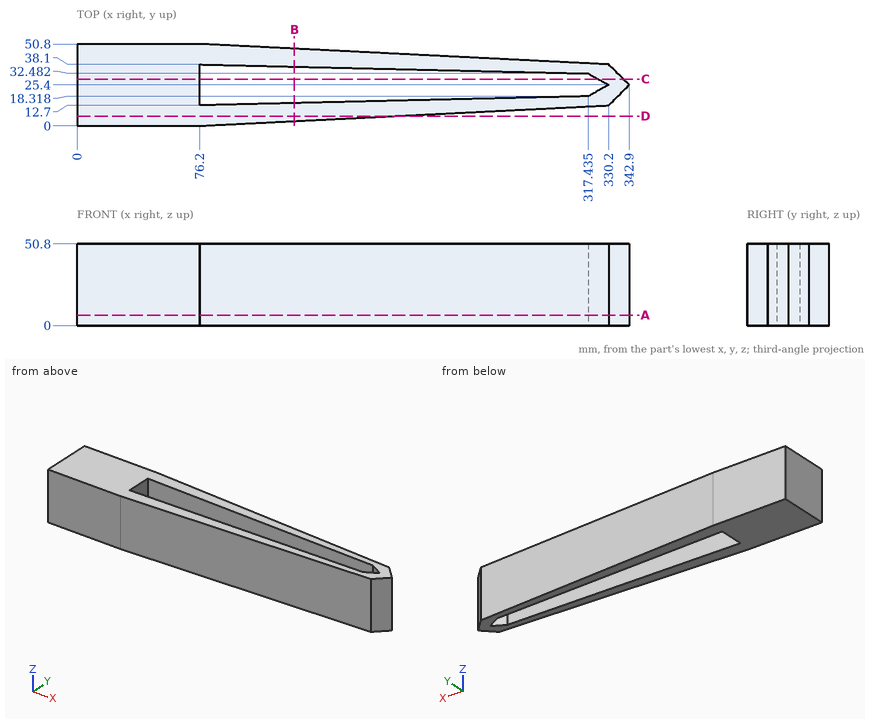
Check sheet for the drawn part. Datum: minimum x, y, z corner. Units: mm. Give positions to 0.01 mm unless a question says otherwise; leave off trailing zeros. Order: outer loops, then holes, each group sorted by start corner. A loop starts at its lowest first (then second) coordinate and runs counter-clockwise, first axis right, second up. Notation, with made-up numbers: (-38.75, 2.5) - (7.25, 2.5) arc R26 ccw to (7.25, 38.5) - close; hole circle Ø5 at (71, 44.5). An arc over 180 degrees is marked (long way). Answer as a JSON object with one key per item and string values.
(1) Cross-section at D-D (y = 6). Record the cut outline in (x, z).
Report:
{"outline": "(0, 0) - (196.2, 0) - (196.2, 50.8) - (0, 50.8) - close"}
(2) Cross-section at C-C (y = 29). Record the cut outline in (x, z).
Report:
{"outline": "(0, 0) - (76.2, 0) - (76.2, 50.8) - (0, 50.8) - close; (323.71, 0) - (339.3, 0) - (339.3, 50.8) - (323.71, 50.8) - close"}
(3) Cross-section at A-A (z = 6.5). Record the cut outline in (x, y) (1 decimal).
Report:
{"outline": "(0, 0) - (76.2, 0) - (330.2, 12.7) - (342.9, 25.4) - (330.2, 38.1) - (76.2, 50.8) - (0, 50.8) - close; hole (76.2, 12.7) - (317.4, 18.3) - (330.2, 25.4) - (317.4, 32.5) - (76.2, 38.1) - close"}
(4) Material ranges on line 1 (X direction, y = 24.5, z = 2) (1 decimal); line 2 (Y direction, x = 100.5, z = 12.5) (1 decimal); line 3 (X direction, y = 25, z = 29.5), recorded low to high.
Report:
{"line 1": "0 to 76.2, 328.6 to 342", "line 2": "1.2 to 13.3, 37.5 to 49.6", "line 3": "0 to 76.2, 329.48 to 342.5"}
(5) Cross-section at B-B (x = 135). Record the cut outline in (y, z), then the cut area to 3 significant figures.
Report:
{"outline": "(2.94, 0) - (14.07, 0) - (14.07, 50.8) - (2.94, 50.8) - close; (36.73, 0) - (47.86, 0) - (47.86, 50.8) - (36.73, 50.8) - close", "area": "1,130 mm^2"}
(6) Depth check by flat-ended pin: pin 1 Ø12 at (y, z) = (29.5, 27.5) entering from +X; pin 2 Ø3 at (x, z) = (177, 43.5) entering from +Y (3 decimals); pin 3 Ø12 at (x, y) = (163.5, 29.5) entering from +Z. Enter the tip coordinate at first touch or a pass-through.
Report:
{"pin 1": "x = 342.9", "pin 2": "y = 45.835", "pin 3": "through"}
